For this review, take the finished solid that the model builds, in its own axes (mm). Coordinates: 2 decimals unless noted, no trailing zeros. Order: outer loops, then holes, each group sorted by start corner. A loop starts at its lowest first (then second) coordinate and runs counter-clockwise, first axis right, second up. Notation, with made-up numbers: M 15.5,53.25 L 37.5,53.25 A22 ccw 37.5,67.25 Z; hole C -32.75,85 d7. An arc over 180 degrees is marked long. Use one line per item in the form item = value. Start each with the question number.
```python
from build123d import *

# Parameters (mm, degrees)
F0_R            = 50
F0_R_2          = 5
F1_DEPTH        = 5
F2_R            = 5
F3_DEPTH        = 25
F3_COPIES_COUNT = 6


# Not quite as in the source:
# - a pattern or mirror of a feature is missing from the dataset's text; its kind, count and spacing are read off the source's solid


with BuildPart() as f1:
    # F0 (on Top) → F1 (new body)
    with BuildSketch(Plane.XY):
        Circle(F0_R)
        Circle(F0_R_2, mode=Mode.SUBTRACT)
    extrude(amount=F1_DEPTH)

    # F2 (on face) → F3 (cut)
    with BuildSketch(Plane.XY.offset(5)):
        with Locations((0, 30)):
            Circle(F2_R)
    f3 = extrude(amount=-F3_DEPTH, mode=Mode.SUBTRACT)

    # F3_copies: F3 ×6 about axis
    f3_copies_axis = Axis((0, 0, 0), (0, 0, 1))
    for i in range(1, F3_COPIES_COUNT):
        add(f3.rotate(f3_copies_axis, i * 360 / F3_COPIES_COUNT), mode=Mode.SUBTRACT)


solid = f1.part
```
1. Consider section D-D, the plane x = -27. Write out the cut boundary in (y, z), plus the area to 3 significant figures.
2. Consider section C-C, the plane y = -15. Write out the cut boundary in (x, z).
3. Consider section A-A, the plane x = 0. Write out the cut boundary in (y, z), plus the area to 3 significant figures.
4. For pin 1 Ø3 at (y, z) = (6.5, 4.5) entering from -X; pin 2 Ø2 at (x, z) = (-11.5, 2.5) entering from -Y; pin 3 Ø3 at (x, z) = (-8.5, 1) entering from -Y, all flat-tipped, find the tip position at first contact; note any pin that passes through.
5. The part is to be moulded in two halves that separate along Y. For faces 1 (the cylindrical face through (-21.21, -13.5, 2.54)), 2 (the flat face through (10, 1, 5)), 3 (the cylindrical face through (47.69, 15.02, 2.46)), say which applies: pulls with the +Y half, pulls with the -Y half, needs draft (parallel to the pull), parting line crosses it, or undercut.
6. Consider section B-B, the plane y = 0. Write out the cut boundary in (x, z), plus the area to 3 significant figures.
7. To check wall thickness, follow line 1 (Y direction, x = 0, z = 2.9); line 2 (X direction, y = -11, z = 3.35) (3 decimals); line 3 (Y direction, x = 22, z = 4). State the ranges of each line that lie inside material, in increasing order.
Answers follow:
q1.outline = M -42.08,0 L -19.9,0 L -19.9,5 L -42.08,5 Z; M -10.1,0 L 10.1,0 L 10.1,5 L -10.1,5 Z; M 19.9,0 L 42.08,0 L 42.08,5 L 19.9,5 Z
q1.area = 323 mm²
q2.outline = M -47.7,0 L -30.98,0 L -30.98,5 L -47.7,5 Z; M -20.98,0 L 20.98,0 L 20.98,5 L -20.98,5 Z; M 30.98,0 L 47.7,0 L 47.7,5 L 30.98,5 Z
q3.outline = M -50,0 L -35,0 L -35,5 L -50,5 Z; M -25,0 L -5,0 L -5,5 L -25,5 Z; M 5,0 L 25,0 L 25,5 L 5,5 Z; M 35,0 L 50,0 L 50,5 L 35,5 Z
q3.area = 350 mm²
q4.pin_1 = -49.75
q4.pin_2 = -48.89
q4.pin_3 = -49.51
q5.face_1 = undercut
q5.face_2 = needs draft
q5.face_3 = parting line crosses it
q6.outline = M -50,0 L -5,0 L -5,5 L -50,5 Z; M 5,0 L 50,0 L 50,5 L 5,5 Z
q6.area = 450 mm²
q7.line_1 = -50 to -35, -25 to -5, 5 to 25, 35 to 50
q7.line_2 = -48.775 to -28.981, -22.981 to 22.981, 28.981 to 48.775
q7.line_3 = -44.9 to -18.03, -11.97 to 11.97, 18.03 to 44.9
